The model under review builds one solid part; all positions refer to its coordinate system, in mm. Coordinates: 2 decimals unless noted, no trailing zeros. Loops run counter-clockwise (first coordinate to the right, second up) from the corner with the lowest first, then second, coordinate; pieces in that order, holes last. Notation, with made-up numbers: (45.5, 66.25) - (99.5, 66.25) arc R20 cw to (99.5, 86.25) - close; hole circle Ø2 at (-35.75, 53.25). An arc over 180 degrees is marked (long way). Answer in a Markdown table with one row per item. Add a question column.
(1) Mouldability with a two-part tool opening along Z and no side actions: class faces 1 (the flat face through (31.739, 5, -27)), 2 (the cylindrical face through (-18.75, 4.93, 9.01)), 3 (the flat face through (-81.05, 4.93, -41.74)) as +Z half, -Z half, draft (parallel to the pull), parting line (faces both ways), or undercut.
(2) We need section D-D on z = -4. Write out the cut boundary in (x, y), plus the area to 3 significant figures.
(3) We need section A-A on z = -60. Write out the cut boundary in (x, y).
(4) We need section B-B on y = 1.75. Give the number of separate pieces and of enclosed holes in the cut face, plus the area to 3 significant figures.
(5) We need section C-C on z = 9. Write out the cut boundary in (x, y).
(6) For line 1 along Z through (x, y) = (2, 9); line 2 along X through (y, z) = (3.5, -59.5); line 3 along Z through (x, y) = (-5, 5.5), list the stretches that pass through material, from the lowest coordinate up.
from build123d import *

# Parameters (mm, degrees)
SKETCH_1_R      = 1.525
SKETCH_1_R_2    = 2.525
EXTRUDE_1_DEPTH = 10


with BuildPart() as part:
    # 草图1 → 凸台-拉伸1 (new body)
    with BuildSketch(Plane(origin=(0, 0, 0), x_dir=(1, 0, 0), z_dir=(0, 1, 0))):
        Polygon((-63.358095006, 31.840104985), (-63.358095006, -17.203623146), (31.738923617, -17.203623146), (31.738923617, 72.796376854), (-33.261076383, 72.796376854), (-98.261076383, 72.796376854), (-98.261076383, 51.371029704), align=None)
        with Locations(Location((-27.261076383, 36.796376854, 0), (0, 0, 270))):
            Circle(SKETCH_1_R, mode=Mode.SUBTRACT)
        with Locations(Location((-51.261076383, 36.796376854, 0), (0, 0, 270))):
            Circle(SKETCH_1_R, mode=Mode.SUBTRACT)
        with Locations(Location((-51.261076383, 6.796376854, 0), (0, 0, 270))):
            Circle(SKETCH_1_R, mode=Mode.SUBTRACT)
        with Locations(Location((-27.261076383, 6.796376854, 0), (0, 0, 270))):
            Circle(SKETCH_1_R, mode=Mode.SUBTRACT)
        with Locations(Location((-20.261076383, -9.203623146, 0), (0, 0, 270))):
            Circle(SKETCH_1_R, mode=Mode.SUBTRACT)
        with Locations(Location((14.738923617, -9.203623146, 0), (0, 0, 270))):
            Circle(SKETCH_1_R, mode=Mode.SUBTRACT)
        with Locations(Location((-6.261076383, 6.796376854, 0), (0, 0, 270))):
            Circle(SKETCH_1_R, mode=Mode.SUBTRACT)
        with Locations(Location((1.73657712, 6.796376854, 0), (0, 0, 270))):
            Circle(SKETCH_1_R, mode=Mode.SUBTRACT)
        with Locations(Location((9.73657712, 6.796376854, 0), (0, 0, 270))):
            Circle(SKETCH_1_R, mode=Mode.SUBTRACT)
        with Locations(Location((17.738923617, 6.796376854, 0), (0, 0, 270))):
            Circle(SKETCH_1_R, mode=Mode.SUBTRACT)
        with Locations(Location((-6.261076383, 16.796376854, 0), (0, 0, 270))):
            Circle(SKETCH_1_R, mode=Mode.SUBTRACT)
        with Locations(Location((1.73657712, 16.796376854, 0), (0, 0, 270))):
            Circle(SKETCH_1_R, mode=Mode.SUBTRACT)
        with Locations(Location((9.73657712, 16.796376854, 0), (0, 0, 270))):
            Circle(SKETCH_1_R, mode=Mode.SUBTRACT)
        with Locations(Location((17.738923617, 16.796376854, 0), (0, 0, 270))):
            Circle(SKETCH_1_R, mode=Mode.SUBTRACT)
        with Locations(Location((-84.594304082, 60.796376854, 0), (0, 0, 270))):
            Circle(SKETCH_1_R_2, mode=Mode.SUBTRACT)
        with Locations(Location((-60.594304082, 60.796376854, 0), (0, 0, 270))):
            Circle(SKETCH_1_R_2, mode=Mode.SUBTRACT)
        with Locations(Location((-6.261076383, 26.796376854, 0), (0, 0, 270))):
            Circle(SKETCH_1_R, mode=Mode.SUBTRACT)
        with Locations(Location((1.73657712, 26.796376854, 0), (0, 0, 270))):
            Circle(SKETCH_1_R, mode=Mode.SUBTRACT)
        with Locations(Location((9.73657712, 26.796376854, 0), (0, 0, 270))):
            Circle(SKETCH_1_R, mode=Mode.SUBTRACT)
        with Locations(Location((17.738923617, 26.796376854, 0), (0, 0, 270))):
            Circle(SKETCH_1_R, mode=Mode.SUBTRACT)
        with Locations(Location((-6.261076383, 36.796376854, 0), (0, 0, 270))):
            Circle(SKETCH_1_R, mode=Mode.SUBTRACT)
        with Locations(Location((1.73657712, 36.796376854, 0), (0, 0, 270))):
            Circle(SKETCH_1_R, mode=Mode.SUBTRACT)
        with Locations(Location((9.73657712, 36.796376854, 0), (0, 0, 270))):
            Circle(SKETCH_1_R, mode=Mode.SUBTRACT)
        with Locations(Location((17.738923617, 36.796376854, 0), (0, 0, 270))):
            Circle(SKETCH_1_R, mode=Mode.SUBTRACT)
        with Locations(Location((-5.927848684, 60.796376854, 0), (0, 0, 270))):
            Circle(SKETCH_1_R_2, mode=Mode.SUBTRACT)
        with Locations(Location((18.072151316, 60.796376854, 0), (0, 0, 270))):
            Circle(SKETCH_1_R_2, mode=Mode.SUBTRACT)
    extrude(amount=EXTRUDE_1_DEPTH)


solid = part.part
Outcome:
| question | item | result |
|---|---|---|
| 1 | face 1 | draft |
| 1 | face 2 | undercut |
| 1 | face 3 | +Z half |
| 2 | outline | (-63.36, 0) - (31.74, 0) - (31.74, 10) - (-63.36, 10) - close |
| 2 | area | 951 mm² |
| 3 | outline | (-98.26, 0) - (-86.99, 0) - (-86.99, 10) - (-98.26, 10) - close; (-82.2, 0) - (-62.99, 0) - (-62.99, 10) - (-82.2, 10) - close; (-58.2, 0) - (-8.32, 0) - (-8.32, 10) - (-58.2, 10) - close; (-3.53, 0) - (15.68, 0) - (15.68, 10) - (-3.53, 10) - close; (20.47, 0) - (31.74, 0) - (31.74, 10) - (20.47, 10) - close |
| 4 | separate pieces | 1 |
| 4 | enclosed holes | 26 |
| 4 | area | 9,410 mm² |
| 5 | outline | (-63.36, 0) - (-21.77, 0) - (-21.77, 10) - (-63.36, 10) - close; (-18.75, 0) - (13.23, 0) - (13.23, 10) - (-18.75, 10) - close; (16.25, 0) - (31.74, 0) - (31.74, 10) - (16.25, 10) - close |
| 6 | line 1 | -72.8 to -38.3, -35.29 to -28.3, -25.29 to -18.3, -15.29 to -8.3, -5.29 to 17.2 |
| 6 | line 2 | -98.26 to -86.76, -82.43 to -62.76, -58.43 to -8.09, -3.76 to 15.91, 20.24 to 31.74 |
| 6 | line 3 | -72.8 to -63.14, -58.45 to -37.65, -35.94 to -27.65, -25.94 to -17.65, -15.94 to -7.65, -5.94 to 17.2 |
